Part model, mm, in its own coordinate system. A direction names the side the tool comes from. Round coordinates to 2 decimals unless told otherwise and drop trailing zeros. Loops run counter-clockwise (first coordinate to the right, second up) from the corner with the lowest first, then second, coordinate; pieces in that order, holes last.
(1) Cut at A-A on z = 191.5. List the corners of the cut face in (x, y), then the cut area to 3 significant figures.
(2) Mould opens along X. For faces 1 (the face through (-7.5, 39.4, 15.1)), 2 (the face through (0, 40.386, 13)), 3 (the face through (-38.136, 38.196, 12.657)), 4 (the face through (33.433, 10.529, 167.98)) say: +X half, -X half, draft (parallel to the pull), parting line (faces both ways), or undercut.
(3) Cut at C-C on x = 13.5. List the corners of the cut face in (y, z).
(4) Tool access for faces 5 (the face through (1.38, -6.2, -7.89)), 6 (the face through (-17, -31.3, 32.766)), 7 (the face through (-7.5, -39.4, 15.1)), 8 (the face through (-39.361, -6.986, 9.067)), 9 (the face through (39.38, -6.76, 16.22)): list every direction of +Z, -Z, +X, -X, +Y, -Y with a clear straight run to the whole face (end or side of a thin tool).
(5) Probe probe 1 along Y at (x, z) = (0, 169) (3 decimals); probe 2 along Y at (x, z) = (0, 110.5) (3 decimals); probe 3 along Z at (x, y) = (24.5, -16.5). List the from-to ranges inside material, lowest first.
(6) Cut at D-D on z = 53. List the corners of the cut face in (x, y) (3 decimals).
(7) Cut at B-B on y = -10.5. List the corners of the cut face in (x, z).
(8) Flat gauge pins, fed straight in: pin 1 (1.6 mm diameter, centred on x = 0, y = 25.019, fed in from -Z); pin 2 (2 mm diameter, centred on x = 25, y = -0.5, fed in from +Z); pin 3 (5 mm diameter, centred on x = -16, z = 169, fed in from -Y). Where does each tip first touch, or does it go through?
from build123d import *

# Parameters (mm, degrees)
SKETCH1_R            = 35.306
SKETCH1_R_2          = 1.016
BASE_EXTRUDE_DEPTH   = 165.1
SKETCH2_R            = 38.608
BOSS_EXTRUDE1_DEPTH  = 32.766
SKETCH3_R            = 6.35
BOSS_EXTRUDE2_DEPTH  = 43.942
SKETCH4_R            = 17.4625
BOSS_EXTRUDE3_DEPTH  = 8.382
SKETCH7_R            = 7.874
BOSS_EXTRUDE5_DEPTH  = 40.386
SKETCH9_R            = 7.62
BOSS_EXTRUDE7_DEPTH  = 80.772
SKETCH11_R           = 7.874
BOSS_EXTRUDE8_DEPTH  = 40.386
SKETCH12_R           = 7.874
BOSS_EXTRUDE10_DEPTH = 80.772
SKETCH13_R           = 9.398
BOSS_EXTRUDE11_DEPTH = 53.975
FILLET1_R            = 6.35
SKETCH14_R           = 6.35
BOSS_EXTRUDE12_DEPTH = 16.002
SKETCH15_R           = 35.052
SKETCH15_R_2         = 1.016
SKETCH15_R_3         = 0.889
BOSS_EXTRUDE13_DEPTH = 5.842


with BuildPart() as part:
    # Sketch1 → Base-Extrude (new body)
    with BuildSketch(Plane.XY):
        Circle(SKETCH1_R)
        with Locations((25.019, 0)):
            Circle(SKETCH1_R_2, mode=Mode.SUBTRACT)
        with Locations((0, 25.019)):
            Circle(SKETCH1_R_2, mode=Mode.SUBTRACT)
        with Locations((-25.019, 0)):
            Circle(SKETCH1_R_2, mode=Mode.SUBTRACT)
        with Locations((0, -25.019)):
            Circle(SKETCH1_R_2, mode=Mode.SUBTRACT)
    extrude(amount=BASE_EXTRUDE_DEPTH)

    # Sketch2 → Boss-Extrude1 (add)
    with BuildSketch(Plane(origin=(0, 0, 0), x_dir=(-1, 0, 0), z_dir=(0, 0, -1))):
        Circle(SKETCH2_R)
    extrude(amount=-BOSS_EXTRUDE1_DEPTH)

    # Sketch3 → Boss-Extrude2 (add)
    with BuildSketch(Plane.XY.offset(165.1)):
        Circle(SKETCH3_R)
    extrude(amount=BOSS_EXTRUDE2_DEPTH)

    # Sketch4 → Boss-Extrude3 (add)
    with BuildSketch(Plane.XY.offset(165.1)):
        Circle(SKETCH4_R)
    extrude(amount=BOSS_EXTRUDE3_DEPTH)

    # Sketch7 → Boss-Extrude5 (add)
    with BuildSketch(Plane(origin=(0, 0, 0), x_dir=(0, 0, -1), z_dir=(1, 0, 0))):
        with Locations((-12.7, 0)):
            Circle(SKETCH7_R)
    extrude(amount=-BOSS_EXTRUDE5_DEPTH)

    # Sketch9 → Boss-Extrude7 (add)
    with BuildSketch(Plane.ZY.offset(40.386)):
        with Locations((12.7, 0)):
            Circle(SKETCH9_R)
    extrude(amount=-BOSS_EXTRUDE7_DEPTH)

    # Sketch11 → Boss-Extrude8 (add)
    with BuildSketch(Plane(origin=(0, 0, 0), x_dir=(-1, 0, 0), z_dir=(0, 1, 0))):
        with Locations((0, 12.7)):
            Circle(SKETCH11_R)
    extrude(amount=BOSS_EXTRUDE8_DEPTH)

    # Sketch12 → Boss-Extrude10 (add)
    with BuildSketch(Plane(origin=(0, 40.386, 0), x_dir=(-1, 0, 0), z_dir=(0, 1, 0))):
        with Locations((0, 12.7)):
            Circle(SKETCH12_R)
    extrude(amount=-BOSS_EXTRUDE10_DEPTH)

    # Sketch13 → Boss-Extrude11 (add)
    with BuildSketch(Plane(origin=(0, 0, 0), x_dir=(0, 0, 1), z_dir=(-0.707106781, 0.707106781, 0))):
        with Locations((12.7, 0)):
            Circle(SKETCH13_R)
    extrude(amount=BOSS_EXTRUDE11_DEPTH)

    # Fillet1
    fillet1_edges = [part.edges().sort_by_distance(p)[0] for p in [
        (-38.166088515, 38.166088515, 3.302),
    ]]
    fillet(fillet1_edges, radius=FILLET1_R)

    # Sketch14 → Boss-Extrude12 (add)
    with BuildSketch(Plane(origin=(0, 0, 0), x_dir=(-1, 0, 0), z_dir=(0, 0, -1))):
        Circle(SKETCH14_R)
    extrude(amount=BOSS_EXTRUDE12_DEPTH)

    # Sketch15 → Boss-Extrude13 (add)
    with BuildSketch(Plane.XY.offset(165.1)):
        Circle(SKETCH15_R)
        with Locations((25.019, 0)):
            Circle(SKETCH15_R_2, mode=Mode.SUBTRACT)
        with Locations((0, 25.019)):
            Circle(SKETCH15_R_3, mode=Mode.SUBTRACT)
        with Locations((0, -25.019)):
            Circle(SKETCH15_R_2, mode=Mode.SUBTRACT)
        with Locations((-25.019, 0)):
            Circle(SKETCH15_R_3, mode=Mode.SUBTRACT)
    extrude(amount=BOSS_EXTRUDE13_DEPTH)


solid = part.part
Final values:
1. outline: circle Ø12.7 at (0, 0)
1. area: 127 mm2
2. face 1: undercut
2. face 2: draft
2. face 3: -X half
2. face 4: parting line
3. outline: (-36.17, 0) - (36.17, 0) - (36.17, 32.77) - (32.62, 32.77) - (32.62, 165.1) - (32.35, 165.1) - (32.35, 170.94) - (11.08, 170.94) - (11.08, 173.48) - (-11.08, 173.48) - (-11.08, 170.94) - (-32.35, 170.94) - (-32.35, 165.1) - (-32.62, 165.1) - (-32.62, 32.77) - (-36.17, 32.77) - close
4. face 5: -Z
4. face 6: +Z
4. face 7: -Y
4. face 8: -X
4. face 9: +X
5. probe 1: y = -35.052 to -26.035, -24.003 to 24.13, 25.908 to 35.052
5. probe 2: y = -35.306 to -26.035, -24.003 to 24.003, 26.035 to 35.306
5. probe 3: z = 0 to 170.94
6. outline: circle Ø70.612 at (0, 0); hole circle Ø2.032 at (-25.019, 0); hole circle Ø2.032 at (0, -25.019); hole circle Ø2.032 at (0, 25.019); hole circle Ø2.032 at (25.019, 0)
7. outline: (-37.15, 0) - (37.15, 0) - (37.15, 32.77) - (33.71, 32.77) - (33.71, 165.1) - (33.44, 165.1) - (33.44, 170.94) - (13.95, 170.94) - (13.95, 173.48) - (-13.95, 173.48) - (-13.95, 170.94) - (-33.44, 170.94) - (-33.44, 165.1) - (-33.71, 165.1) - (-33.71, 32.77) - (-37.15, 32.77) - close
8. pin 1: stops at z = 0
8. pin 2: stops at z = 170.94
8. pin 3: stops at y = -32.35
